Check sheet for the modelled part. Datum: model origin and axes. Units: mm. Face numbers are marked on the shaded views. Round coordinates to 2 decimals unless told otherwise and drop trailing zeros. Loops run counter-clockwise (first coordinate to the right, second up) from the corner with the lowest first, then second, coordinate; pieces in that order, holes last. Notation, with made-up numbers: (46.5, 66.5) -> (101.5, 66.5) arc R16 cw to (101.5, 81.5) -> close; hole circle Ø8 at (-40, 55.5). An arc over 180 degrees is marked (long way). One line per item, written item: value. Start each with the question number.
1. Release check for a two-part mould opening along X. For the marked faces 1, 2 and 3 record: +X half, -X half, draft (parallel to the pull), parting line (faces both ways), or undercut.
2. Cross-section at D-D on y = 16.5. Record the cut outline in (x, z).
3. Material ranges on L1, parallel to X at y = 23.5, z = 4.5; L2, parallel to X at y = 12, z = 0.75, recorded low to high.
4. Cross-section at B-B on y = 24. Record the cut outline in (x, z), then the cut area to 3 significant figures.
5. Cross-section at A-A on z = 11.5. Record the cut outline in (x, y).
6. Go/stop test with flat-tipped pins: pin 1 (3 mm diameter, centred on y = 10.5, z = -4.5, fed in from -X); pin 2 (9 mm diameter, centred on y = 10.5, z = -4, fed in from -X); pin 3 (4 mm diameter, centred on y = 26, z = 3, fed in from -X). Record where each tip stops, or that it passes through.
7. Cross-section at C-C on z = 1.25. Record the cut outline in (x, y).
from build123d import *

# Parameters (mm, degrees)
SKETCH_1_W      = 30
SKETCH_1_H      = 30
EXTRUDE_1_DEPTH = 30


with BuildPart() as part:
    # 스케치1 → 보스-돌출1 (new body)
    with BuildSketch(Plane(origin=(0, 0, 0), x_dir=(1, 0, 0), z_dir=(0, 1, 0))):
        Rectangle(SKETCH_1_W, SKETCH_1_H)
    extrude(amount=EXTRUDE_1_DEPTH)

    # 스케치2 → 회전1 (revolve)
    with BuildSketch(Plane.XY):
        with BuildLine():
            Line((-17.5, 15), (-4.5, 15))
            ThreePointArc((-4.5, 15), (-11, 21.5), (-17.5, 15))
        make_face()
    revolve(axis=Axis((-17.5, 15, 0), (1, 0, 0)))


solid = part.part
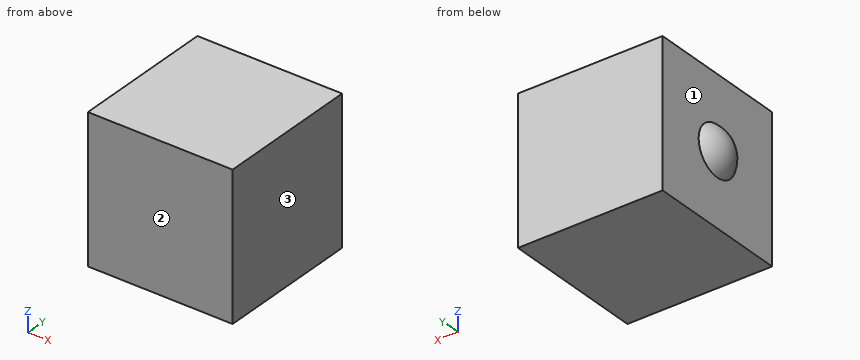
Taken from the geometry:
1. face 1: -X half
1. face 2: draft
1. face 3: +X half
2. outline: (-15, -15) -> (15, -15) -> (15, 15) -> (-15, 15) -> (-15, 4.9) arc R6.32 ccw to (-15, -4.9) -> close
3. L1: x = -15 to 15
3. L2: x = -16.72 to 15
4. outline: (-15, -15) -> (15, -15) -> (15, 15) -> (-15, 15) -> close
4. area: 900 mm2
5. outline: (-15, 0) -> (15, 0) -> (15, 30) -> (-15, 30) -> close
6. pin 1: stops at x = -15.31
6. pin 2: stops at x = -17.32
6. pin 3: stops at x = -15
7. outline: (-15, 0) -> (15, 0) -> (15, 30) -> (-15, 30) -> (-15, 19.97) arc R6.38 ccw to (-15, 10.03) -> close
